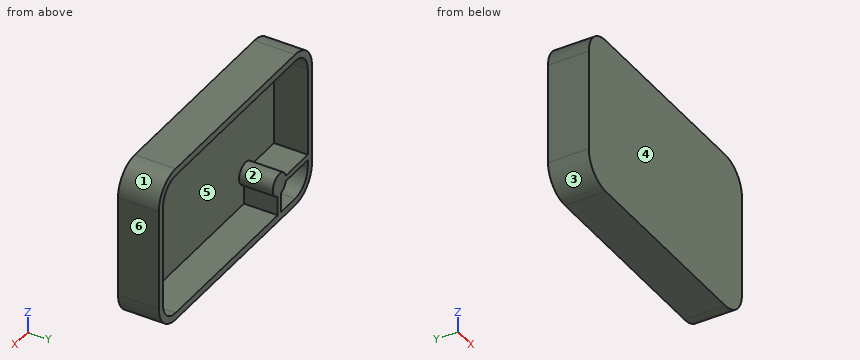
```python
from build123d import *

# Parameters (mm, degrees)
BOSS_EXTRUDE1_DEPTH = 18.542
SHELL1_T            = -3.175
BOSS_EXTRUDE2_REACH = 139.638
SKETCH2_R           = 5.019286765
RIB1_REACH          = 139.638
SKETCH3_WALLS_W     = 293.719610529
SKETCH3_WALLS_H     = 2.54
SKETCH3_WALLS_W_2   = 2.54
SKETCH3_WALLS_H_2   = 286.179283193


with BuildPart() as part:
    # Sketch1 → Boss-Extrude1 (new body)
    with BuildSketch(Plane(origin=(0, 0, 0), x_dir=(1, 0, 0), z_dir=(0, 1, 0))):
        with BuildLine():
            Line((12.7, 0), (103.254058747, 0))
            ThreePointArc((103.254058747, 0), (112.234314868, 3.719743879), (115.954058747, 12.7))
            Line((115.954058747, 12.7), (115.954058747, 59.098953312))
            ThreePointArc((115.954058747, 59.098953312), (112.234314868, 68.079209433), (103.254058747, 71.798953312))
            Line((103.254058747, 71.798953312), (12.7, 71.798953312))
            ThreePointArc((12.7, 71.798953312), (3.719743879, 68.079209433), (0, 59.098953312))
            Line((0, 59.098953312), (0, 12.7))
            ThreePointArc((0, 12.7), (3.719743879, 3.719743879), (12.7, 0))
        make_face()
    extrude(amount=-BOSS_EXTRUDE1_DEPTH)

    # Shell1
    shell1_openings = [part.faces().sort_by_distance(p)[0] for p in [
        (57.977029373, 0, -35.899476656),
    ]]
    offset(amount=SHELL1_T, openings=shell1_openings, kind=Kind.INTERSECTION)

    # Sketch2 → Boss-Extrude2 (add, up to next)
    with BuildSketch(Plane(origin=(0, 0, 0), x_dir=(1, 0, 0), z_dir=(0, 1, 0)), mode=Mode.PRIVATE) as boss_extrude2_sk1:
        with Locations(Location((24.637750849, 54.7015298, 0), (0, 0, 270))):
            Circle(SKETCH2_R)
    boss_extrude2_tool1 = extrude(boss_extrude2_sk1.sketch, amount=-BOSS_EXTRUDE2_REACH, mode=Mode.PRIVATE) - part.part
    add(boss_extrude2_tool1.solids().sort_by_distance((24.637751, 0, -54.70153))[0])

    # Sketch3 walls → Rib1 (add, up to next)
    with BuildSketch(Plane(origin=(0, 0, 0), x_dir=(1, 0, 0), z_dir=(0, 1, 0)), mode=Mode.PRIVATE) as rib1_sk1:
        with Locations((11.396732042, 54.7015298)):
            Rectangle(SKETCH3_WALLS_W, SKETCH3_WALLS_H)
    rib1_tool1 = extrude(rib1_sk1.sketch, amount=-RIB1_REACH, mode=Mode.PRIVATE) - part.part
    # Sketch3 walls → Rib1 (add, up to next)
    with BuildSketch(Plane(origin=(0, 0, 0), x_dir=(1, 0, 0), z_dir=(0, 1, 0)), mode=Mode.PRIVATE) as rib1_sk2:
        with Locations((24.637750849, 64.172384939)):
            Rectangle(SKETCH3_WALLS_W_2, SKETCH3_WALLS_H_2)
    rib1_tool2 = extrude(rib1_sk2.sketch, amount=-RIB1_REACH, mode=Mode.PRIVATE) - part.part
    add(rib1_tool1.solids().sort_by_distance((11.396732042, 0, -54.7015298))[0])
    add(rib1_tool2.solids().sort_by_distance((24.637750849, 0, -64.172384939))[0])


solid = part.part
```
CAD build for the part. Positions are in the model's coordinates, mm. Face numbers are marked on the shaded views. A direction names the side the tool comes from. Coordinates: 2 decimals unless noted, no trailing zeros. Write each loop counter-clockwise with the first axis right and the second up, starting at its lowest first coordinate (ties: lowest second). Pieces come first, ordered by that corner, then holes.
(1) Flat gauge pins, fed straight in: pin 1 (4.5 mm diameter, centred on x = 12.5, y = -10.5, fed in from -Z); pin 2 (3 mm diameter, centred on y = -8.5, z = -7.5, fed in from -X); pin 3 (7.5 mm diameter, centred on y = -11.5, z = -64, fed in from -X); pin 4 (8 mm diameter, centred on x = 102.5, z = -49, fed in from +Y). Where does each tip first touch, or does it go through?
(2) 3-axis set-ups, long thin cutter, end or side, ignore diameter. For the marked faces 5 and 6: which of +Z, -Z, +X, -X, +Y, -Y reach the whole face in a straight line?
(3) Cut at D-D, the plane z = -52. List the corners of the cut face in (x, y) (1 decimal).
(4) Two-plate mould, pull along X, no slides. Class the marked faces 1, 2, 3 and 4: +X half, -X half, draft (parallel to the pull), parting line (faces both ways), or undercut.
(5) Cut at B-B, the plane z = -40. List the corners of the cut face in (x, y) (3 decimals).
(6) Drill centre lines: probe 1 along Z at (x, y) = (93.5, -15.25) (3 decimals); probe 2 along X at (y, z) = (-2.5, -62); probe 3 along X at (y, z) = (-4.5, -27.5) (3 decimals). Where is each one in solid material? Low to high.
(7) Cut at A-A, the plane y = -10. List the corners of the cut face in (x, z) (3 decimals), and give its area (3 significant figures).
(8) Cut at C-C, the plane x = 69. List the corners of the cut face in (y, z) (3 decimals).
Geometry says:
1. pin 1: stops at z = -71.8
1. pin 2: stops at x = 0.55
1. pin 3: stops at x = 0.05
1. pin 4: stops at y = -15.37
2. face 5: +Y
2. face 6: +Z, -Z, +X, +Y, -Y
3. outline: (0, -18.5) - (116, -18.5) - (116, 0) - (112.8, 0) - (112.8, -15.4) - (28.9, -15.4) - (28.9, 0) - (20.4, 0) - (20.4, -15.4) - (3.2, -15.4) - (3.2, 0) - (0, 0) - close
4. face 1: +X half
4. face 2: undercut
4. face 3: -X half
4. face 4: draft
5. outline: (0, -18.542) - (115.954, -18.542) - (115.954, 0) - (112.779, 0) - (112.779, -15.367) - (3.175, -15.367) - (3.175, 0) - (0, 0) - close
6. probe 1: z = -71.799 to -68.624, -3.175 to 0
6. probe 2: x = 0.34 to 3.63, 23.37 to 25.91, 112.33 to 115.62
6. probe 3: x = 0 to 3.175, 112.779 to 115.954
7. outline: (0, -59.099) arc R12.7 ccw to (12.7, -71.799) - (103.254, -71.799) arc R12.7 ccw to (115.954, -59.099) - (115.954, -12.7) arc R12.7 ccw to (103.254, 0) - (12.7, 0) arc R12.7 ccw to (0, -12.7) - close; hole (3.175, -59.099) arc R9.525 ccw to (12.7, -68.624) - (23.368, -68.624) - (23.368, -59.557) arc R5.019 cw to (19.782, -55.972) - (3.175, -55.972) - close; hole (3.175, -53.432) - (19.782, -53.432) arc R5.019 cw (long way) to (25.908, -59.557) - (25.908, -68.624) - (103.254, -68.624) arc R9.525 ccw to (112.779, -59.099) - (112.779, -12.7) arc R9.525 ccw to (103.254, -3.175) - (12.7, -3.175) arc R9.525 ccw to (3.175, -12.7) - close
7. area: 1,240 mm2
8. outline: (-18.542, -71.799) - (0, -71.799) - (0, -68.624) - (-15.367, -68.624) - (-15.367, -3.175) - (0, -3.175) - (0, 0) - (-18.542, 0) - close
